Geometry check sheet. Reference: the model listing, model coordinates, mm. Coordinates: 2 decimals unless noted, no trailing zeros. Write each loop counter-clockwise with the first axis right and the second up, starting at its lowest first coordinate (ties: lowest second). Pieces come first, ordered by that corner, then holes. Notation, with made-up numbers: M -39.5,37.5 L -27.5,37.5 A6 ccw -27.5,43.5 Z; hole C 39.25,-0.75 d9. An arc over 180 degrees is marked long. Write each question's results on one line, items separated by ' | '.
```python
from build123d import *

# Parameters (mm, degrees)
F0_W       = 406.4
F0_H       = 19.05
F1_DEPTH   = 1727.2
F2_W       = 12.7
F2_H       = 6.35
F1_FACE1_W = 406.4
F1_FACE1_H = 19.05
F3_DEPTH   = 1727.201
F4_W       = 12.7
F4_H       = 6.35
F5_DEPTH   = 1727.201


with BuildPart() as f1:
    # F0 (on Top) → F1 (new body)
    with BuildSketch(Plane.XY):
        with Locations((0, -9.525)):
            Rectangle(F0_W, F0_H)
    extrude(amount=F1_DEPTH)

    # F2 (on face) + F1_face1 (on face) → F3 (cut, through all)
    with BuildSketch(Plane.XY.offset(1727.2)):
        with Locations((196.85, -3.175)):
            Rectangle(F2_W, F2_H)
    with BuildSketch(Plane(origin=(0, -9.525, 0), x_dir=(1, 0, 0), z_dir=(0, 0, -1))):
        Rectangle(F1_FACE1_W, F1_FACE1_H)
    extrude(amount=-F3_DEPTH, dir=(0, 0, 1), mode=Mode.SUBTRACT)

    # F4 (on face) → F5 (cut, through all)
    with BuildSketch(Plane.XY.offset(1727.2)):
        with Locations((-196.85, -3.175)):
            Rectangle(F4_W, F4_H)
    extrude(amount=-F5_DEPTH, mode=Mode.SUBTRACT)


solid = f1.part
```
Q1. Depth check by flat-ended pin: P1, Ø5, axis at y = -3.5, z = 1227.5, coming from the +X side; P2, Ø10, axis at x = 199.5, z = 670, coming from the +Y side; P3, Ø1.9, axis at y = -3.5, z = 939.5, coming from the -X side. Enter the tip coordinate at first touch or a pass-through.
Geometry check:
P1: stops at x = 190.5 | P2: stops at y = -6.35 | P3: stops at x = -190.5
Q2. Scan line: probe 1 along X at (y, z) = (-3.5, 166). Record every from-to range of solid material in increasing order.
Geometry check:
probe 1: x = -190.5 to 190.5
Q3. Sectioned sample at A-A on z = 1053.5. Record the cut outline in (x, y).
Geometry check:
outline: M -203.2,-19.05 L 203.2,-19.05 L 203.2,-6.35 L 190.5,-6.35 L 190.5,0 L -190.5,0 L -190.5,-6.35 L -203.2,-6.35 Z
